from build123d import *


with BuildPart() as part:
    # Sketch → Revolution (revolve)
    with BuildSketch(Plane.XZ):
        Polygon((6, 16), (6, -16), (11, -16), (11, -12), (10, -12), (10, -11), (11, -11), (11, 11), (10, 11), (10, 12), (11, 12), (11, 16), align=None)
    revolve(axis=Axis((0, 0, 0), (0, 0, 1)))


solid = part.part
Check sheet for the modelled part. Datum: model origin and axes. Units: mm. A direction names the side the tool comes from. Round coordinates to 2 decimals unless told otherwise and drop trailing zeros. Loops run counter-clockwise (first coordinate to the right, second up) from the corner with the lowest first, then second, coordinate; pieces in that order, holes last. Notation, with made-up numbers: M 28.5,-11 L 83.5,-11 A20 ccw 83.5,14 Z; hole C 78.5,35 d3. An arc over 180 degrees is marked long. One line per item, written item: value.
(1) Sectioned sample at C-C, the plane z = -5. Record the cut outline in (x, y).
Computed values:
outline: C 0,0 d22; hole C 0,0 d12
(2) Depth check by flat-ended pin: pin 1 Ø1.5 at (y, z) = (-8.5, 8.5) entering from -X; pin 2 Ø1 at (y, z) = (4, 1.5) entering from -X. Enter the tip coordinate at first touch or a pass-through.
Computed values:
pin 1: stops at x = -7.81
pin 2: stops at x = -10.43
(3) Access from +Z, -Z, +X, -X, +Y, -Y to the whole of each face (thin tool, end or side, straight path). Record for faces 4 (the face through (-2, -10, 12)), 5 (the face through (-2.38, -10.74, 0.15)).
Computed values:
face 4: none
face 5: +Z, -Z
(4) Sectioned sample at A-A, the plane x = 0. Record the cut outline in (y, z).
Computed values:
outline: M -11,-16 L -6,-16 L -6,16 L -11,16 L -11,12 L -10,12 L -10,11 L -11,11 L -11,-11 L -10,-11 L -10,-12 L -11,-12 Z; M 6,-16 L 11,-16 L 11,-12 L 10,-12 L 10,-11 L 11,-11 L 11,11 L 10,11 L 10,12 L 11,12 L 11,16 L 6,16 Z
(5) Thickness scan on line 1 (Z direction, x = 6, y = -8.25); line 2 (Y direction, x = 0, z = -1.5); line 3 (Y direction, x = -2.75, z = 12.5). Record the ranges inside material, lowest first.
Computed values:
line 1: z = -16 to -12, -11 to 11, 12 to 16
line 2: y = -11 to -6, 6 to 11
line 3: y = -10.65 to -5.33, 5.33 to 10.65
(6) Sectioned sample at D-D, the plane y = 9.5. Record the cut outline in (x, z), then the cut area to 3 significant figures.
Computed values:
outline: M -5.55,-16 L 5.55,-16 L 5.55,-12 L 3.12,-12 L 3.12,-11 L 5.55,-11 L 5.55,11 L 3.12,11 L 3.12,12 L 5.55,12 L 5.55,16 L -5.55,16 L -5.55,12 L -3.12,12 L -3.12,11 L -5.55,11 L -5.55,-11 L -3.12,-11 L -3.12,-12 L -5.55,-12 Z
area: 345 mm^2
(7) Release check for a two-part mould opening along Z. For faces 1 (the face through (2, -10, 11)), 2 (the face through (5, -5, 16)), 3 (the face through (-2.38, -10.74, 14.03)) record: +Z half, -Z half, draft (parallel to the pull), parting line (faces both ways), or undercut.
Computed values:
face 1: undercut
face 2: +Z half
face 3: draft
